Part model, mm, in its own coordinate system. Face numbers are marked on the shaded views. A direction names the side the tool comes from. Coordinates: 2 decimals unless noted, no trailing zeros. Order: outer loops, then holes, each group sorted by start corner. A loop starts at its lowest first (then second) coordinate and runs counter-clockwise, first axis right, second up. Notation, with made-up numbers: (21.25, 66.25) - (39.25, 66.25) arc R22 cw to (39.25, 105.25) - close; hole circle Ø8 at (37.25, -23.5). An arc over 180 degrees is marked (long way). Use a Markdown table: item, result. Add a question column.
1) Drop flat-ended pins along their axis: P1, Ø5, axis at x = 16, z = 102, coming from the +Y side; P2, Ø7.5, axis at x = 81.77, y = 81.77, coming from the -Z side; P3, Ø15.5, axis at x = 16.5, z = -6.5, coming from the +Y side; P4, Ø4, axis at x = 59, y = 25, coming from the +Z side. Give the stop position or say it passes through.
2) Wall check: L1, parallel to Z at x = 14, y = -3.8; L2, parallel to Y at x = 21, z = 25.5; L3, parallel to Z at x = 36.5, y = 33. Give the ranges that are in metal, low to high. Write a range as [from, to].
3) Saw through at C-C on z = -7. List the corners of the cut face in (x, y), then the cut area to 3 significant figures.
4) Tool access for the marked faces 1 and 2: list every direction of +Z, -Z, +X, -X, +Y, -Y with a clear straight run to the whole face (end or side of a thin tool).
5) Saw through at B-B on z = 110. List the corners of the cut face in (x, y), then the cut area to 3 significant figures.
6) Saw through at A-A on y = 63. List the corners of the cut face in (x, z), then the cut area to 3 significant figures.
7) Saw through at D-D on y = 73. List the corners of the cut face in (x, z).
```python
from build123d import *

# Parameters (mm, degrees)
CYLINDER_R        = 2.78
CYLINDER_DEPTH    = 10
CYLINDER001_R     = 2.78
CYLINDER001_DEPTH = 10
EXTRUDE002_DEPTH  = 6
CYLINDER003_R     = 2.78
CYLINDER003_DEPTH = 10
CYLINDER002_R     = 2.78
CYLINDER002_DEPTH = 10
SKETCH001_W       = 90
SKETCH001_H       = 6
EXTRUDE001_DEPTH  = 209.55
SKETCH_R          = 3.25
SKETCH_R_2        = 18
EXTRUDE_DEPTH     = 10


with BuildPart() as cylinder:
    # Cylinder → Cylinder (new body)
    with BuildSketch(Plane(origin=(14, 2, -7), x_dir=(1, 0, 0), z_dir=(0, -1, 0))):
        Circle(CYLINDER_R)
    extrude(amount=CYLINDER_DEPTH)


with BuildPart() as cylinder001:
    # Cylinder001 → Cylinder001 (new body)
    with BuildSketch(Plane(origin=(76, 2, -7), x_dir=(1, 0, 0), z_dir=(0, -1, 0))):
        Circle(CYLINDER001_R)
    extrude(amount=CYLINDER001_DEPTH)


with BuildPart() as cut001:
    # Sketch002 (on Face1 of Extrude001) → Extrude002 (new body)
    with BuildSketch(Plane.XZ.offset(6)):
        with BuildLine():
            ThreePointArc((0, 0), (14, -14), (28, 0))
            Line((0, 0), (28, 0))
        make_face()
        with BuildLine():
            ThreePointArc((62, 0), (76, -14), (90, 0))
            Line((62, 0), (90, 0))
        make_face()
    extrude(amount=-EXTRUDE002_DEPTH)

    # Cut: cut Cylinder001
    add(cylinder001.part, mode=Mode.SUBTRACT)

    # Cut001: cut Cylinder
    add(cylinder.part, mode=Mode.SUBTRACT)


with BuildPart() as cylinder003:
    # Cylinder003 → Cylinder003 (new body)
    with BuildSketch(Plane(origin=(80, 2, 110), x_dir=(1, 0, 0), z_dir=(0, -1, 0))):
        Circle(CYLINDER003_R)
    extrude(amount=CYLINDER003_DEPTH)


with BuildPart() as cylinder002:
    # Cylinder002 → Cylinder002 (new body)
    with BuildSketch(Plane(origin=(10, 2, 110), x_dir=(1, 0, 0), z_dir=(0, -1, 0))):
        Circle(CYLINDER002_R)
    extrude(amount=CYLINDER002_DEPTH)


with BuildPart() as cut003:
    # Sketch001 (on Sketch) → Extrude001 (new body)
    with BuildSketch(Plane.XY):
        with Locations((45, -3)):
            Rectangle(SKETCH001_W, SKETCH001_H)
    extrude(amount=EXTRUDE001_DEPTH)

    # Cut002: cut Cylinder002
    add(cylinder002.part, mode=Mode.SUBTRACT)

    # Cut003: cut Cylinder003
    add(cylinder003.part, mode=Mode.SUBTRACT)


with BuildPart() as fusion:
    # Sketch → Extrude (new body)
    with BuildSketch(Plane.XY):
        Polygon((0, 0), (0, 90), (90, 90), (90, 0), (90, -6), (0, -6), align=None)
        with Locations((8.230447, 81.769553)):
            Circle(SKETCH_R, mode=Mode.SUBTRACT)
        with Locations((81.769553, 81.769553)):
            Circle(SKETCH_R, mode=Mode.SUBTRACT)
        with Locations((81.769553, 8.230447)):
            Circle(SKETCH_R, mode=Mode.SUBTRACT)
        with Locations((8.230447, 8.230447)):
            Circle(SKETCH_R, mode=Mode.SUBTRACT)
        with Locations((45, 63)):
            Circle(SKETCH_R_2, mode=Mode.SUBTRACT)
    extrude(amount=EXTRUDE_DEPTH)

    # Fusion: union Cut001, Cut003
    add(cut001.part)
    add(cut003.part)


solid = fusion.part
```
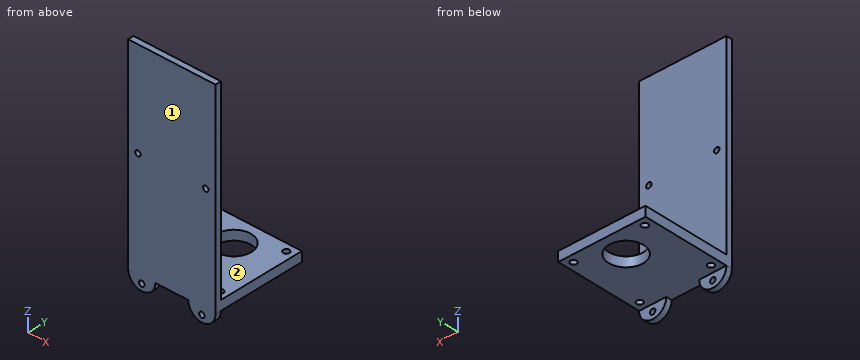
Results are:
| question | item | result |
|---|---|---|
| 1 | P1 | y = 0 |
| 1 | P2 | z = 0 |
| 1 | P3 | y = 90 |
| 1 | P4 | z = 10 |
| 2 | L1 | [-14, -9.78], [-4.22, 209.55] |
| 2 | L2 | [-6, 0] |
| 2 | L3 | [0, 10] |
| 3 | outline | (1.88, -6) - (11.22, -6) - (11.22, 0) - (1.88, 0) - close; (16.78, -6) - (26.12, -6) - (26.12, 0) - (16.78, 0) - close; (63.88, -6) - (73.22, -6) - (73.22, 0) - (63.88, 0) - close; (78.78, -6) - (88.12, -6) - (88.12, 0) - (78.78, 0) - close |
| 3 | area | 224 mm2 |
| 4 | face 1 | +Z, -Z, +X, -X, -Y |
| 4 | face 2 | +Z, +X, -X, +Y |
| 5 | outline | (0, -6) - (7.22, -6) - (7.22, 0) - (0, 0) - close; (12.78, -6) - (77.22, -6) - (77.22, 0) - (12.78, 0) - close; (82.78, -6) - (90, -6) - (90, 0) - (82.78, 0) - close |
| 5 | area | 473 mm2 |
| 6 | outline | (0, 0) - (27, 0) - (27, 10) - (0, 10) - close; (63, 0) - (90, 0) - (90, 10) - (63, 10) - close |
| 6 | area | 540 mm2 |
| 7 | outline | (0, 0) - (30.03, 0) - (30.03, 10) - (0, 10) - close; (59.97, 0) - (90, 0) - (90, 10) - (59.97, 10) - close |
